from build123d import *

# Parameters (mm, degrees)
SKETCH1_W               = 173
SKETCH1_H               = 170
BOSS_EXTRUDE1_DEPTH     = 1.5
SKETCH2_W               = 173
SKETCH2_H               = 41.5
BOSS_EXTRUDE2_DEPTH     = 1.5
SKETCH3_W               = 173
SKETCH3_H               = 41.5
BOSS_EXTRUDE3_DEPTH     = 1.5
SKETCH4_R               = 1.5
CUT_EXTRUDE1_DEPTH      = 1000
CUT_EXTRUDE1_DEPTH_BACK = 1000
SKETCH5_R               = 1.5
CUT_EXTRUDE2_DEPTH      = 5
CUT_EXTRUDE2_DEPTH_BACK = 5


with BuildPart() as part:
    # Sketch1 → Boss-Extrude1 (new body)
    with BuildSketch(Plane(origin=(0, 0, 0), x_dir=(1, 0, 0), z_dir=(0, 1, 0))):
        with Locations((86.5, 85)):
            Rectangle(SKETCH1_W, SKETCH1_H)
    extrude(amount=BOSS_EXTRUDE1_DEPTH)

    # Sketch2 → Boss-Extrude2 (add)
    with BuildSketch(Plane.XY):
        with Locations((86.5, -19.25)):
            Rectangle(SKETCH2_W, SKETCH2_H)
    extrude(amount=BOSS_EXTRUDE2_DEPTH)

    # Sketch3 → Boss-Extrude3 (add)
    with BuildSketch(Plane(origin=(0, 0, -170), x_dir=(-1, 0, 0), z_dir=(0, 0, -1))):
        with Locations((-86.5, -19.25)):
            Rectangle(SKETCH3_W, SKETCH3_H)
    extrude(amount=BOSS_EXTRUDE3_DEPTH)

    # Sketch4 → Cut-Extrude1 (cut, two sides)
    with BuildSketch(Plane(origin=(0, 0, -171.5), x_dir=(-1, 0, 0), z_dir=(0, 0, -1))) as cut_extrude1_sk:
        with Locations((-156.5, -32)):
            Circle(SKETCH4_R)
        with Locations((-16.5, -32)):
            Circle(SKETCH4_R)
    extrude(amount=CUT_EXTRUDE1_DEPTH, mode=Mode.SUBTRACT)
    extrude(cut_extrude1_sk.sketch, amount=-CUT_EXTRUDE1_DEPTH_BACK, mode=Mode.SUBTRACT)

    # Sketch5 → Cut-Extrude2 (cut, two sides)
    with BuildSketch(Plane(origin=(0, 1.5, 0), x_dir=(1, 0, 0), z_dir=(0, 1, 0))) as cut_extrude2_sk:
        with Locations((79, 10)):
            Circle(SKETCH5_R)
        with Locations((79, 160)):
            Circle(SKETCH5_R)
        with Locations((93, 10)):
            Circle(SKETCH5_R)
        with Locations((93, 160)):
            Circle(SKETCH5_R)
    extrude(amount=CUT_EXTRUDE2_DEPTH, mode=Mode.SUBTRACT)
    extrude(cut_extrude2_sk.sketch, amount=-CUT_EXTRUDE2_DEPTH_BACK, mode=Mode.SUBTRACT)


solid = part.part
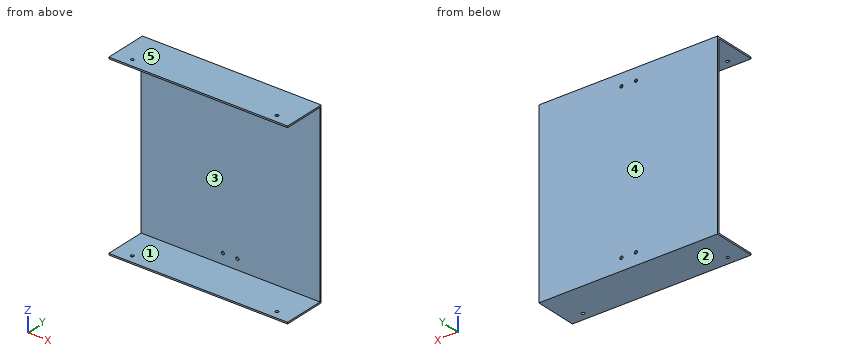
The listing builds one solid part. Answer for the finished solid, in the listing's coordinates (mm). Face numbers are marked on the shaded views. A direction names the side the tool comes from. Round coordinates to 2 decimals unless told otherwise and drop trailing zeros. Write each loop counter-clockwise with the first axis right and the second up, starting at its lowest first coordinate (ties: lowest second). Pieces come first, ordered by that corner, then holes. Notation, with made-up numbers: (39, 13) - (65, 13) arc R17 cw to (65, 23) - close; hole circle Ø7 at (-31.5, -8). An arc over 180 degrees is marked (long way). Use a Markdown table: item, result. Add a question column.
1. For a pull along Z with two mould halves and no side action, classify the marked faces 3, 4 and 5 as +Z half, -Z half, draft (parallel to the pull), parting line (faces both ways), or undercut.
2. Flat-ended cylindrical pins translate along their axes: P1, Ø4, axis at x = 53.5, z = -84, coming from the -Y side; P2, Ø5, axis at x = 156.5, y = -32, coming from the -Z side. Find the tip coordinate at first contact, or state that the pin passes through.
3. The part is cut by section C-C (z = -139.5). Write down the section's boundary in (x, y).
4. The part is cut by section B-B (x = 42). Write down the section's boundary in (y, z), and give its area (4 significant figures).
5. Consider line 1 (Z direction, x = 93, y = 0.35); line 2 (Z direction, x = 121, y = -14.5); line 3 (Y direction, x = 72, z = -116). Determine where each line is inside the solid, lowest interval first.
6. The part is cut by section A-A (y = -18). Write down the section's boundary in (x, z).
7. A tool of negligible diameter and unlimited length cuts with its end or side. For the marked faces 1 and 2, from which of +Z, -Z, +X, -X, +Y, -Y can it reach the whole face along a straight path? Write none if from no direction.
Reported:
| question | item | result |
|---|---|---|
| 1 | face 3 | undercut |
| 1 | face 4 | draft |
| 1 | face 5 | +Z half |
| 2 | P1 | y = 0 |
| 2 | P2 | z = -171.5 |
| 3 | outline | (0, 0) - (173, 0) - (173, 1.5) - (0, 1.5) - close |
| 4 | outline | (-40, -171.5) - (1.5, -171.5) - (1.5, 1.5) - (-40, 1.5) - (-40, 0) - (0, 0) - (0, -170) - (-40, -170) - close |
| 4 | area | 379.5 mm^2 |
| 5 | line 1 | -171.5 to -161.5, -158.5 to -11.5, -8.5 to 1.5 |
| 5 | line 2 | -171.5 to -170, 0 to 1.5 |
| 5 | line 3 | 0 to 1.5 |
| 6 | outline | (0, -171.5) - (173, -171.5) - (173, -170) - (0, -170) - close; (0, 0) - (173, 0) - (173, 1.5) - (0, 1.5) - close |
| 7 | face 1 | +X, -X, -Y |
| 7 | face 2 | -Z, +X, -X, +Y, -Y |
